```python
from build123d import *

# Parameters (mm, degrees)
SKETCH1_W                                         = 60.198
SKETCH1_H                                         = 37.846
BOSS_EXTRUDE1_DEPTH                               = 3.302
FILLET1_R                                         = 3.302
CSK_FOR_4_FLAT_HEAD_MACHINE_SCREW_100_D           = 3.2639
CSK_FOR_4_FLAT_HEAD_MACHINE_SCREW_100_CSINK_D     = 5.715
CSK_FOR_4_FLAT_HEAD_MACHINE_SCREW_100_CSINK_ANGLE = 100


with BuildPart() as part:
    # Sketch1 → Boss-Extrude1 (new body)
    with BuildSketch(Plane(origin=(0, 0, 0), x_dir=(1, 0, 0), z_dir=(0, 1, 0))):
        Rectangle(SKETCH1_W, SKETCH1_H)
    extrude(amount=BOSS_EXTRUDE1_DEPTH)

    # Fillet1
    fillet1_edges = [part.edges().sort_by_distance(p)[0] for p in [
        (30.099, 1.651, 18.923),
        (-30.099, 1.651, 18.923),
        (-30.099, 1.651, -18.923),
        (30.099, 1.651, -18.923),
    ]]
    fillet(fillet1_edges, radius=FILLET1_R)

    # CSK for #4 Flat Head Machine Screw (100)1 (through all)
    with Locations(Plane(origin=(0, 3.302, 0), x_dir=(1, 0, 0), z_dir=(0, 1, 0))):
        with Locations((-26.289, 15.113), (-26.289, -15.113), (26.289, -15.113), (26.289, 15.113)):
            CounterSinkHole(CSK_FOR_4_FLAT_HEAD_MACHINE_SCREW_100_D / 2, CSK_FOR_4_FLAT_HEAD_MACHINE_SCREW_100_CSINK_D / 2, counter_sink_angle=CSK_FOR_4_FLAT_HEAD_MACHINE_SCREW_100_CSINK_ANGLE)


solid = part.part
```
Model file for the job. Use its own axes, mm. Round coordinates to 2 decimals unless told otherwise and drop trailing zeros. Order: outer loops, then holes, each group sorted by start corner. A loop starts at its lowest first (then second) coordinate and runs counter-clockwise, first axis right, second up. Notation, with made-up numbers: (-30, -16) -> (-7, -16) arc R24 ccw to (-7, 21) -> close; hole circle Ø1 at (83.5, 54.5). An arc over 180 degrees is marked (long way). Use one line per item in the form item = value.
Item 1: Pull direction X, two halves, no side cores. Call faces 1 (the face through (0, 2, 18.923)), 2 (the face through (29.16, 1.67, -17.93)), 3 (the face through (-25.086, 1.121, 14.01)): released by +X, released by -X, zero draft, split by the parting line, or undercut.
Returned:
face_1 = zero draft
face_2 = released by +X
face_3 = undercut
Item 2: Drill centre lines: line 1 (X direction, y = 1.4, z = -15); line 2 (X direction, y = 2.6, z = -14); line 3 (Z direction, x = 25, y = 1.9). Where is each one in solid material? Low to high.
Returned:
line_1 = -30.1 to -27.92, -24.66 to 24.66, 27.92 to 30.1
line_2 = -30.1 to -27.98, -24.6 to 24.6, 27.98 to 30.1
line_3 = -18.92 to -16.11, -14.11 to 14.11, 16.11 to 18.92
Item 3: Cut at A-A, the plane y = 0.5. Write the cut outline in (x, z), and give its area (3 significant figures).
Returned:
outline = (-30.1, -15.62) arc R3.3 ccw to (-26.8, -18.92) -> (26.8, -18.92) arc R3.3 ccw to (30.1, -15.62) -> (30.1, 15.62) arc R3.3 ccw to (26.8, 18.92) -> (-26.8, 18.92) arc R3.3 ccw to (-30.1, 15.62) -> close; hole circle Ø3.26 at (-26.29, -15.11); hole circle Ø3.26 at (-26.29, 15.11); hole circle Ø3.26 at (26.29, -15.11); hole circle Ø3.26 at (26.29, 15.11)
area = 2,240 mm^2
